Can you work these out from the model? Positions are in its coordinate system, mm. Face numbers are marked on the shaded views. Coordinates: 2 decimals unless noted, no trailing zeros. Order: outer loops, then holes, each group sorted by start corner. A loop starts at its lowest first (then second) coordinate and runs counter-clockwise, first axis right, second up. Notation, with made-up numbers: (0, 7) -> (13, 7) arc R30 ccw to (13, 39) -> close; hole circle Ø11 at (70, -34). An arc over 180 degrees is marked (long way). Write item = value, one per line.
```python
from build123d import *

# Parameters (mm, degrees)
SKETCH1_R           = 25
SKETCH1_R_2         = 5
BOSS_EXTRUDE1_DEPTH = 10
FILLET1_R           = 1
FILLET2_R           = 1


with BuildPart() as part:
    # Sketch1 → Boss-Extrude1 (new body)
    with BuildSketch(Plane.XY):
        Circle(SKETCH1_R)
        Circle(SKETCH1_R_2, mode=Mode.SUBTRACT)
    extrude(amount=BOSS_EXTRUDE1_DEPTH)

    # Fillet1
    fillet1_edges = [part.edges().sort_by_distance(p)[0] for p in [
        (-25, 0, 0),
        (-5, 0, 0),
        (-5, 0, 10),
    ]]
    fillet(fillet1_edges, radius=FILLET1_R)

    # Fillet2
    fillet2_edges = [part.edges().sort_by_distance(p)[0] for p in [
        (-25, 0, 10),
    ]]
    fillet(fillet2_edges, radius=FILLET2_R)


solid = part.part
```
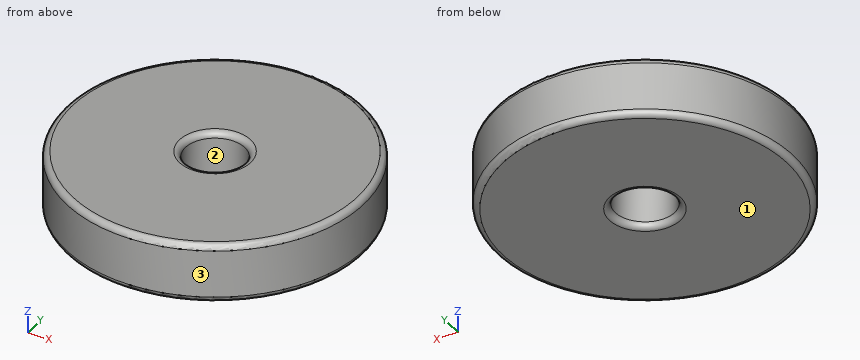
Item 1: If I drill on probe 1 along Y at (x, z) = (0, 7); probe 2 along Y at (x, z) = (1, 3.75); probe 3 along X at (y, z) = (7, 6.5), over which ranges is the centre line in solid material (lowest first)?
A:
probe_1 = -25 to -5, 5 to 25
probe_2 = -24.98 to -4.9, 4.9 to 24.98
probe_3 = -24 to 24
Item 2: I want a section at C-C, the plane z = 5. Please give me the cut outline in (x, y), plus the area to 3 significant figures.
A:
outline = circle Ø50 at (0, 0); hole circle Ø10 at (0, 0)
area = 1,880 mm2
Item 3: I want a section at A-A, the plane y = 0. Please give me the cut outline in (x, z), plus the area to 3 significant figures.
A:
outline = (-25, 1) arc R1 ccw to (-24, 0) -> (-6, 0) arc R1 ccw to (-5, 1) -> (-5, 9) arc R1 ccw to (-6, 10) -> (-24, 10) arc R1 ccw to (-25, 9) -> close; (5, 1) arc R1 ccw to (6, 0) -> (24, 0) arc R1 ccw to (25, 1) -> (25, 9) arc R1 ccw to (24, 10) -> (6, 10) arc R1 ccw to (5, 9) -> close
area = 398 mm2
Item 4: If we mould it in two halves opening along Y, with no side actions, what happens to the marked faces 1, 2 and 3? For each: pulls with the +Y half, pulls with the -Y half, needs draft (parallel to the pull), parting line crosses it, or undercut.
A:
face_1 = needs draft
face_2 = undercut
face_3 = parting line crosses it
Item 5: I'm going to push flat-ended pins straight in: P1, Ø1, axis at y = -10.5, z = 4, coming from the -X side; P2, Ø6, axis at x = -7.5, z = 5, coming from the -Y side; P3, Ø3, axis at y = -9, z = 1, coming from the +X side. Where does each tip first touch, or does it pass through?
A:
P1 = -22.91
P2 = -24.59
P3 = 23.85
